Work out the finished part from the listing and answer in its coordinate system (mm). Round coordinates to 2 decimals unless told otherwise and drop trailing zeros. Order: outer loops, then holes, each group sorted by start corner. A loop starts at its lowest first (then second) coordinate and runs counter-clockwise, first axis right, second up. Notation, with made-up numbers: (-33, 14.25) -> (5, 14.25) arc R36 ccw to (5, 50.25) -> close; hole circle Ø8 at (62, 18.25). An arc over 180 degrees is marked (long way). Use one line per item in the form item = value.
```python
from build123d import *

# Parameters (mm, degrees)
SKETCH1_W           = 47.051856626
SKETCH1_H           = 6.096
SKETCH1_W_2         = 7.62
BOSS_EXTRUDE1_DEPTH = 3.048
CHAMFER2_SIZE       = 3.81


with BuildPart() as part:
    # Sketch1 → Boss-Extrude1 (new body, symmetric)
    with BuildSketch(Plane(origin=(0, 0, 0), x_dir=(0, 0, -1), z_dir=(1, 0, 0))):
        Polygon((45.72, -63.246), (45.72, -16.5735), (38.1, -16.5735), (38.1, -10.4775), (45.72, -10.4775), (45.72, 10.4775), (38.1, 10.4775), (38.1, 16.5735), (45.72, 16.5735), (45.72, 63.246), (-16.571856626, 63.246), (-16.571856626, 16.5735), (-39.096447575, 16.5735), (-43.495856626, 14.0335), (-43.495856626, -14.0335), (-39.096447575, -16.5735), (-16.571856626, -16.5735), (-16.571856626, -63.246), align=None)
        with Locations((14.574071687, -52.578)):
            Rectangle(SKETCH1_W, SKETCH1_H, mode=Mode.SUBTRACT)
        with Locations((14.574071687, 52.578)):
            Rectangle(SKETCH1_W, SKETCH1_H, mode=Mode.SUBTRACT)
        with Locations((7.62, 13.5255)):
            Rectangle(SKETCH1_W_2, SKETCH1_H, mode=Mode.SUBTRACT)
        with Locations((7.62, -13.5255)):
            Rectangle(SKETCH1_W_2, SKETCH1_H, mode=Mode.SUBTRACT)
    extrude(amount=BOSS_EXTRUDE1_DEPTH, both=True)

    # Chamfer2
    chamfer2_edges = [part.edges().sort_by_distance(p)[0] for p in [
        (0, -63.246, -45.72),
        (0, -63.246, 16.571856626),
        (0, 63.246, 16.571856626),
        (0, 63.246, -45.72),
    ]]
    chamfer(chamfer2_edges, length=CHAMFER2_SIZE)


solid = part.part
```
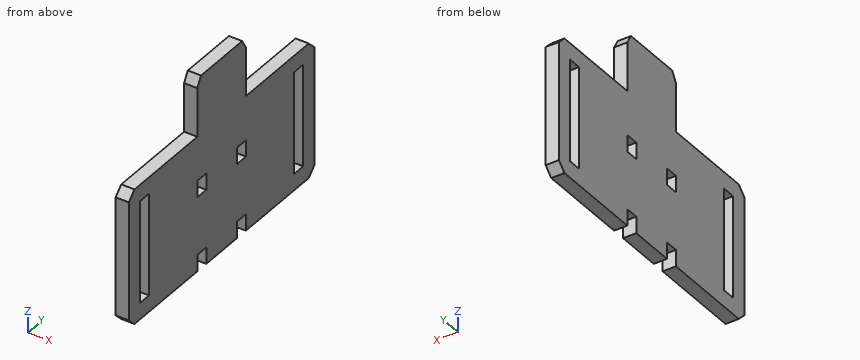
Item 1: The part is cut by section C-C, the plane y = 34. Give the vertices of the cut face in (x, z).
Findings:
outline = (-3.05, -45.72) -> (3.05, -45.72) -> (3.05, 16.57) -> (-3.05, 16.57) -> close
Item 2: The part is cut by section A-A, the plane z = -28. Give the vertices of the cut face in (x, y).
Findings:
outline = (-3.05, -63.25) -> (3.05, -63.25) -> (3.05, -55.63) -> (-3.05, -55.63) -> close; (-3.05, -49.53) -> (3.05, -49.53) -> (3.05, 49.53) -> (-3.05, 49.53) -> close; (-3.05, 55.63) -> (3.05, 55.63) -> (3.05, 63.25) -> (-3.05, 63.25) -> close
Item 3: Flat-ended cylindrical pins translate along their axes: P1, Ø2, axis at x = -1.5, y = -19.5, coming from the +Z side; P2, Ø1.8, axis at x = -0.5, z = -43.5, coming from the -Y side. Find the tip coordinate at first contact, or state that the pin passes through.
Findings:
P1 = 16.57
P2 = -62.56
Item 4: Consider line 1 along Y through (x, z) = (2.5, 3); line 2 along Y through (x, z) = (1.75, -8.5); line 3 along Z through (x, y) = (2, -54.5). Determine where each line is inside the solid, lowest interval first.
Findings:
line_1 = -63.25 to -55.63, -49.53 to 49.53, 55.63 to 63.25
line_2 = -63.25 to -55.63, -49.53 to -16.57, -10.48 to 10.48, 16.57 to 49.53, 55.63 to 63.25
line_3 = -45.72 to -38.1, 8.95 to 16.57
Item 5: The part is cut by section B-B, the plane x = -2. Give the number of separate pieces and of enclosed holes in the cut face, and give its area (3 significant figures).
Findings:
separate_pieces = 1
enclosed_holes = 4
area = 7,970 mm^2
